Design review of the part built by this model. Coordinates are the model's own, in mm. Coordinates: 2 decimals unless noted, no trailing zeros. Loops run counter-clockwise (first coordinate to the right, second up) from the corner with the lowest first, then second, coordinate; pieces in that order, holes last.
Q1. For P1, Ø1.5, axis at x = 1, y = -4.5, coming from the -Z side, flat-tipped, find the tip position at first contact; note if it passes through.
Q2. Add section A-A on y = 0. Give the boundary of the cut face in (x, z).
Q3. Add section C-C on x = -1.25. Give the boundary of the cut face in (y, z).
Q4. Wall thickness on probe 1 along X at (y, z) = (26.5, -2); probe 2 along Z at (x, y) = (2.85, 0); probe 3 along Z at (x, y) = (-0.85, 0): over which ranges is each line inside the solid? List them lowest first.
Autodesk Inventor part; units mm, degrees
ref_plane "YZ Plane" through (0, 0, 0) normal (1, 0, 0) x (0, 1, 0)
ref_plane "XZ Plane" through (0, 0, 0) normal (0, 1, 0) x (-1, 0, 0)
ref_plane "XY Plane" through (0, 0, 0) normal (0, 0, 1) x (1, 0, 0)
sketch "Sketch1" plane through (0, 0, 0) normal (1, 0, 0) x (0, 1, 0)
  circle A0 centre (0, 0) radius 30.25
  circle A1 centre (0, 0) radius 25.4
  dimension "d0" = 60.5
  dimension "d3" = 50.8
extrude "Extrusion1" add sketch "Sketch1" along normal mid plane 8
sketch "Sketch2" plane through (0, 0, 0) normal (1, 0, 0) x (0, 1, 0)
  circle A0 centre (0, 0) radius 28
  dimension "d4" = 56
extrude "Extrusion2" cut sketch "Sketch2" along normal mid plane 5
fillet "Fillet1" radius 1 2 edges at (-4, -30.25, 0) (4, -30.25, 0)
properties part number "Rubber Wheel Cap"
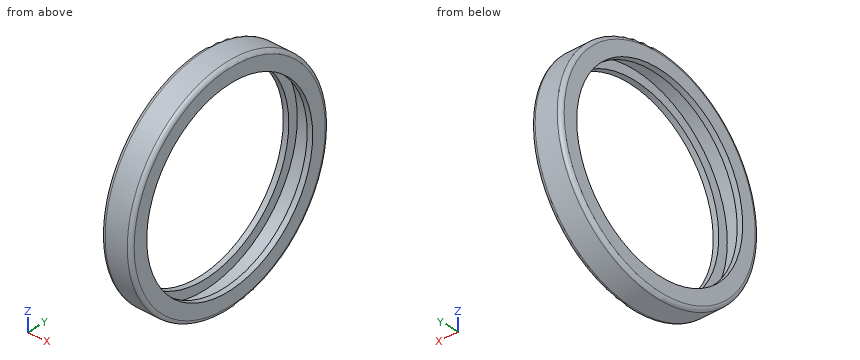
Entries:
1. P1: stops at z = -30.02
2. outline: (-4, -29.25) arc R1 ccw to (-3, -30.25) - (3, -30.25) arc R1 ccw to (4, -29.25) - (4, -25.4) - (2.5, -25.4) - (2.5, -28) - (-2.5, -28) - (-2.5, -25.4) - (-4, -25.4) - close; (-4, 25.4) - (-2.5, 25.4) - (-2.5, 28) - (2.5, 28) - (2.5, 25.4) - (4, 25.4) - (4, 29.25) arc R1 ccw to (3, 30.25) - (-3, 30.25) arc R1 ccw to (-4, 29.25) - close
3. outline: circle Ø60.5 at (0, 0); hole circle Ø56 at (0, 0)
4. probe 1: x = -4 to -2.5, 2.5 to 4
4. probe 2: z = -30.25 to -25.4, 25.4 to 30.25
4. probe 3: z = -30.25 to -28, 28 to 30.25
